Design review of the part built by this model. Coordinates are the model's own, in mm. A direction names the side the tool comes from. Round coordinates to 2 decimals unless told otherwise and drop trailing zeros. Order: outer loops, then holes, each group sorted by start corner. A loop starts at its lowest first (then second) coordinate and runs counter-clockwise, first axis right, second up. Notation, with made-up numbers: M -31.75,12 L -11.75,12 A7 cw -11.75,25 Z; hole C -4.5,-5 d6. An arc over 180 degrees is marked long. Write item = value, one per line. Start each with the question number.
```python
from build123d import *

# Parameters (mm, degrees)
MAIN_DEPTH          = 4
ESQUISSE2_R         = 2.5
BOSS_EXTRUDE1_DEPTH = 1.8


with BuildPart() as part:
    # Esquisse1 → Main (new body)
    with BuildSketch(Plane.XY):
        with BuildLine():
            Line((-4.375785644, 4.25), (-6.426543071, 6.300757427))
            ThreePointArc((-6.426543071, 6.300757427), (-3.48519606, 8.297795395), (0, 9))
            Line((0, 9), (30, 6))
            ThreePointArc((30, 6), (35.9926952, 0.295980134), (30.591239576, -5.970798587))
            Line((30.591239576, -5.970798587), (0, -9))
            ThreePointArc((0, -9), (-3.48519606, -8.297795395), (-6.426543071, -6.300757427))
            Line((-6.426543071, -6.300757427), (-4.375785644, -4.25))
            ThreePointArc((-4.375785644, -4.25), (0, -6.1), (4.375785644, -4.25))
            Line((4.375785644, -4.25), (17.31559729, -2.78215714))
            ThreePointArc((17.31559729, -2.78215714), (19.8, 0), (17.31559729, 2.78215714))
            Line((17.31559729, 2.78215714), (4.375785644, 4.25))
            ThreePointArc((4.375785644, 4.25), (0, 6.1), (-4.375785644, 4.25))
        make_face()
        with BuildLine():
            Line((23.5, 3.25), (30, 3.25))
            ThreePointArc((30, 3.25), (33.25, 0), (30, -3.25))
            Line((30, -3.25), (23.5, -3.25))
            ThreePointArc((23.5, -3.25), (20.25, 0), (23.5, 3.25))
        make_face(mode=Mode.SUBTRACT)
    extrude(amount=MAIN_DEPTH)

    # Esquisse2 → Boss-Extrude1 (add)
    with BuildSketch(Plane(origin=(0, 0, 4), x_dir=(-1, 0, 0), z_dir=(0, 0, -1))):
        with BuildLine():
            Line((0, -9), (-13.303143835, -7.682697966))
            ThreePointArc((-13.303143835, -7.682697966), (-20.25000193, -0.006506175), (-13.303143835, 7.669685617))
            Line((-13.303143835, 7.669685617), (0, 9))
            ThreePointArc((0, 9), (3.48519606, 8.297795395), (6.426543071, 6.300757427))
            Line((6.426543071, 6.300757427), (6.426543071, -6.300757427))
            ThreePointArc((6.426543071, -6.300757427), (3.48519606, -8.297795395), (0, -9))
        make_face()
        Circle(ESQUISSE2_R, mode=Mode.SUBTRACT)
    extrude(amount=BOSS_EXTRUDE1_DEPTH)


solid = part.part
```
(1) Consider section B-B, the plane z = 3.6. Write out the cut boundary in (x, y).
(2) Consider section A-A, the plane z = 1.6. Write out the cut boundary in (x, y), then the cut area to 3 significant figures.
(3) Draft analysis for pull direction X (two halves, no side actions). For faces 1 (the face through (10, 0, 4)), 2 (the face through (14.79, 7.52, 1.97)), 3 (the face through (10.936, 3.506, 1.085)), 4 (the face through (27, 3.25, 2)), state which applies: pulls with the +X half, pulls with the -X half, needs draft (parallel to the pull), parting line crosses it, or undercut.
(4) For line 1 along Y through (x, z) = (0, 3.35); line 2 along Z through (x, y) = (17, 2); line 3 along Y through (x, z) = (23.5, 2.6), list the stretches that pass through material, from the lowest coordinate up. Write a range as [from, to].
(5) Insertion check: pin 1 (1 mm diameter, centred on y = -3, z = 2, fed in from +X); pin 2 (2 mm diameter, centred on x = 28.5, z = 2.5, fed in from -Y); pin 3 (6 mm diameter, centred on x = 0, y = 0, fed in from -Z); pin 4 (3 mm diameter, centred on x = 29, y = -1.5, fed in from +Z). Each pin has a flat end and moves straight along its axis. Give the tip position at first contact, or say it passes through.
(6) Consider section C-C, the plane x = 25. Write out the cut boundary in (y, z).
(7) For faces 5 (the face through (-5.387, 5.261, 1.085)), 6 (the face through (4, 0, 2.2)), 7 (the face through (33.25, 0.07, 1.97)), list the 3-axis set-ups (+Z, -Z, +X, -X, +Y, -Y) from which the entire face can be reached by the end or side of a thin tool; tool diameter is ignored.
(8) Consider section D-D, the plane y = -0.75. Write out the cut boundary in (x, z).
Completed:
q1.outline = M -6.43,-6.3 A9 ccw 0,-9 L 30.59,-5.97 A6 ccw 30,6 L 0,9 A9 ccw -6.43,6.3 Z; hole C 0,0 d5; hole M 23.5,-3.25 L 30,-3.25 A3.25 ccw 30,3.25 L 23.5,3.25 A3.25 ccw Z
q2.outline = M -6.43,-6.3 A9 ccw 0,-9 L 30.59,-5.97 A6 ccw 30,6 L 0,9 A9 ccw -6.43,6.3 L -4.38,4.25 A6.1 cw 4.38,4.25 L 17.32,2.78 A2.8 cw 17.32,-2.78 L 4.38,-4.25 A6.1 cw -4.38,-4.25 Z; hole M 23.5,-3.25 L 30,-3.25 A3.25 ccw 30,3.25 L 23.5,3.25 A3.25 ccw Z
q2.area = 317 mm2
q3.face_1 = needs draft
q3.face_2 = pulls with the +X half
q3.face_3 = pulls with the -X half
q3.face_4 = undercut
q4.line_1 = [-9, -2.5], [2.5, 9]
q4.line_2 = [2.2, 4]
q4.line_3 = [-6.67, -3.25], [3.25, 6.65]
q5.pin_1 = 35.45
q5.pin_2 = -6.28
q5.pin_3 = 2.2
q5.pin_4 = through
q6.outline = M -6.52,0 L -3.25,0 L -3.25,4 L -6.52,4 Z; M 3.25,0 L 6.5,0 L 6.5,4 L 3.25,4 Z
q7.face_5 = -Z, -X
q7.face_6 = -Z
q7.face_7 = +Z, -Z
q8.outline = M -6.43,2.2 L -2.38,2.2 L -2.38,4 L -6.43,4 Z; M 2.38,2.2 L 19.7,2.2 L 19.7,0 L 20.34,0 L 20.34,4 L 2.38,4 Z; M 33.16,0 L 35.95,0 L 35.95,4 L 33.16,4 Z
